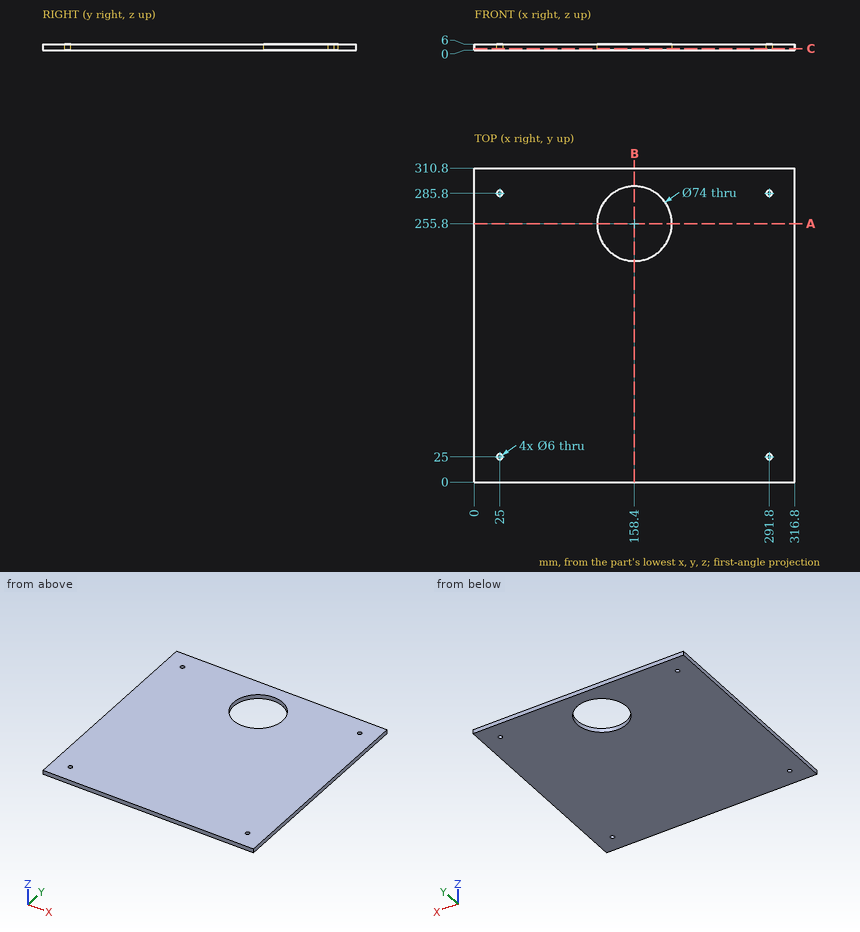
Source: three-view drawing plus pictorial views. Frame: mm from the lowest corner of the part. Round coordinates to 2 decimals unless told otherwise and drop trailing zeros. Loops run counter-clockwise (first coordinate to the right, second up) from the corner with the lowest first, then second, coordinate; pieces in that order, holes last. Notation, with made-up numbers: (12.5, 10) -> (64.5, 10) arc R25 ccw to (64.5, 31) -> close; hole circle Ø10 at (76.25, 5.5). An arc over 180 degrees is marked (long way). Use one line per item in the form item = value.
Item 1: Material intervals for probe 1 along Y at (x, z) = (291.8, 2.6); probe 2 along X at (y, z) = (285.8, 4.5); probe 3 along Y at (x, z) = (290, 4), sorted ascending.
Evaluation:
probe_1 = 0 to 22, 28 to 282.8, 288.8 to 310.8
probe_2 = 0 to 22, 28 to 136.74, 180.06 to 288.8, 294.8 to 316.8
probe_3 = 0 to 22.6, 27.4 to 283.4, 288.2 to 310.8
Item 2: Cut plane B-B on x = 158.4. Output: boundary loops of the cut face in (y, z).
Evaluation:
outline = (0, 0) -> (218.8, 0) -> (218.8, 6) -> (0, 6) -> close; (292.8, 0) -> (310.8, 0) -> (310.8, 6) -> (292.8, 6) -> close
Item 3: Cut plane A-A on y = 255.8. Output: boundary loops of the cut face in (x, z), then the cut area to 3 significant figures.
Evaluation:
outline = (0, 0) -> (121.4, 0) -> (121.4, 6) -> (0, 6) -> close; (195.4, 0) -> (316.8, 0) -> (316.8, 6) -> (195.4, 6) -> close
area = 1,460 mm2
Item 4: Contact query for a flat-ended pin moving along its axis: pin 1 Ø5.5 at (x, y) = (291.8, 285.8) entering from +Z. Output: stop coordinate, or through.
Evaluation:
pin_1 = through
Item 5: Cut plane C-C on z = 1.4. Output: boundary loops of the cut face in (x, y), then the cut area to 3 significant figures.
Evaluation:
outline = (0, 0) -> (316.8, 0) -> (316.8, 310.8) -> (0, 310.8) -> close; hole circle Ø6 at (25, 25); hole circle Ø6 at (25, 285.8); hole circle Ø74 at (158.4, 255.8); hole circle Ø6 at (291.8, 25); hole circle Ø6 at (291.8, 285.8)
area = 94,000 mm2
